Check sheet for the modelled part. Datum: model origin and axes. Units: mm. A direction names the side the tool comes from. Round coordinates to 2 decimals unless told otherwise and drop trailing zeros. Write each loop counter-clockwise with the first axis right and the second up, starting at its lowest first coordinate (ties: lowest second). Pieces come first, ordered by that corner, then holes. Notation, with made-up numbers: M -25.5,-40 L -11.5,-40 A8 cw -11.5,-29 Z; hole C 86.25,43 d8. An arc over 180 degrees is marked long. Put each result on its own line as item: value.
```python
from build123d import *

# Parameters (mm, degrees)
F1_R     = 1.5499996566
F1_R_2   = 4.15
F1_R_3   = 10.975
F2_DEPTH = 15
F3_R     = 1.5499996566
F3_R_2   = 10.975
F3_R_3   = 4.15
F3_R_4   = 5
F4_DEPTH = 8
F5_SIZE  = 0.5


# Not quite as in the source:
# - a feature names something its author has since deleted; it is built from what else it names


with BuildPart() as f2:
    # F1 (on offset) → F2 (new body)
    with BuildSketch(Plane.XZ.offset(7.5)):
        with BuildLine():
            ThreePointArc((-16.6892397333, 5.7083826769), (-18.3305665894, 4.8749174948), (-20.1713586703, 4.8647896648))
            ThreePointArc((-20.1713586703, 4.8647896648), (-26.2950827169, -0.0072979827), (-20.1713596113, -4.879386813))
            ThreePointArc((-20.1713596113, -4.879386813), (-18.3305675322, -4.8895149984), (-16.6892408371, -5.7229804975))
            ThreePointArc((-16.6892408371, -5.7229804975), (-14.008426037, -7.1768258733), (-10.9702112996, -7.4408061354))
            ThreePointArc((-10.9702112996, -7.4408061354), (-6.8485397196, -7.8126278343), (-3.2303605207, -9.8214103693))
            ThreePointArc((-3.2303605207, -9.8214103693), (7.2785660743, -12.855093715), (16.3833205976, -6.7933928076))
            ThreePointArc((16.3833205976, -6.7933928076), (18.1382514389, -5.2406931628), (20.4617514792, -4.9373682419))
            ThreePointArc((20.4617514792, -4.9373682419), (26.2950863861, -0.0073004118), (20.4617519197, 4.9227679396))
            ThreePointArc((20.4617519197, 4.9227679396), (18.1382519066, 5.2260930681), (16.383321204, 6.7787928697))
            ThreePointArc((16.383321204, 6.7787928697), (7.2785667206, 12.8404946682), (-3.2303604104, 9.8068115182))
            ThreePointArc((-3.2303604104, 9.8068115182), (-6.8485396319, 7.7980290238), (-10.970211216, 7.4262073712))
            ThreePointArc((-10.970211216, 7.4262073712), (-14.0084253044, 7.1622273392), (-16.6892397333, 5.7083826769))
        make_face()
        with Locations((21.2950848365, -0.0073001884)):
            Circle(F1_R, mode=Mode.SUBTRACT)
        with Locations((-21.2950828407, -0.0072984656)):
            Circle(F1_R, mode=Mode.SUBTRACT)
        with Locations((-11.8549144411, -0.0072993771)):
            Circle(F1_R_2, mode=Mode.SUBTRACT)
        with Locations((5.2950859535, -0.0072994735)):
            Circle(F1_R_3, mode=Mode.SUBTRACT)
    extrude(amount=-F2_DEPTH)

    # F3 (on face) → F4 (join)
    with BuildSketch(Plane(origin=(0, 7.5, 0), x_dir=(-1, 0, 0), z_dir=(0, 1, 0))):
        with BuildLine():
            ThreePointArc((10.970211216, 7.4262073712), (6.8485396319, 7.7980290238), (3.2303604104, 9.8068115182))
            ThreePointArc((3.2303604104, 9.8068115182), (-7.2785667206, 12.8404946682), (-16.383321204, 6.7787928697))
            ThreePointArc((-16.383321204, 6.7787928697), (-18.1382519066, 5.2260930681), (-20.4617519197, 4.9227679396))
            ThreePointArc((-20.4617519197, 4.9227679396), (-26.2950863861, -0.0073004118), (-20.4617514792, -4.9373682419))
            ThreePointArc((-20.4617514792, -4.9373682419), (-18.1382514389, -5.2406931628), (-16.3833205976, -6.7933928076))
            ThreePointArc((-16.3833205976, -6.7933928076), (-7.2785660743, -12.855093715), (3.2303605207, -9.8214103693))
            ThreePointArc((3.2303605207, -9.8214103693), (6.8485397196, -7.8126278343), (10.9702112996, -7.4408061354))
            ThreePointArc((10.9702112996, -7.4408061354), (14.008426037, -7.1768258733), (16.6892408371, -5.7229804975))
            ThreePointArc((16.6892408371, -5.7229804975), (18.3305675322, -4.8895149984), (20.1713596113, -4.879386813))
            ThreePointArc((20.1713596113, -4.879386813), (26.2950827169, -0.0072979827), (20.1713586703, 4.8647896648))
            ThreePointArc((20.1713586703, 4.8647896648), (18.3305665894, 4.8749174948), (16.6892397333, 5.7083826769))
            ThreePointArc((16.6892397333, 5.7083826769), (14.0084253044, 7.1622273392), (10.970211216, 7.4262073712))
        make_face()
        with Locations((-21.2950848365, -0.0073001884)):
            Circle(F3_R, mode=Mode.SUBTRACT)
        with Locations((-5.2950859535, -0.0072994735)):
            Circle(F3_R_2, mode=Mode.SUBTRACT)
        with Locations((11.8549144411, -0.0072993771)):
            Circle(F3_R_3, mode=Mode.SUBTRACT)
        with Locations((21.2950828407, -0.0072984656)):
            Circle(F3_R, mode=Mode.SUBTRACT)
        with Locations((-5.2950859535, -0.0072994735)):
            Circle(F3_R_2)
        with Locations((-5.2950859535, -0.0072994735)):
            Circle(F3_R_4, mode=Mode.SUBTRACT)
    extrude(amount=-F4_DEPTH)

    # F5
    f5_edges = [f2.edges().sort_by_distance(p)[0] for p in [
        (-6.84854, -7.5, 7.798029),
        (7.278567, -7.5, 12.840495),
        (18.138252, -7.5, 5.226093),
        (26.295086, -7.5, -0.0073),
        (18.138251, -7.5, -5.240693),
        (7.278566, -7.5, -12.855094),
        (-6.84854, -7.5, -7.812628),
        (-14.008426, -7.5, -7.176826),
        (-18.330568, -7.5, -4.889515),
        (-26.295083, -7.5, -0.007298),
        (-18.330567, -7.5, 4.874917),
        (-14.008425, -7.5, 7.162227),
        (-5.679914, -7.5, -0.007299),
        (-22.845082, -7.5, -0.007298),
        (19.745085, -7.5, -0.0073),
        (7.278567, 7.5, 12.840495),
        (-22.845082, 7.5, -0.007298),
        (10.295086, 7.5, -0.007299),
        (19.745085, 7.5, -0.0073),
        (-16.004914, -7.5, -0.007299),
        (-6.84854, 7.5, 7.798029),
        (-14.008425, 7.5, 7.162227),
        (-18.330567, 7.5, 4.874917),
        (-26.295083, 7.5, -0.007298),
        (-18.330568, 7.5, -4.889515),
        (-14.008426, 7.5, -7.176826),
        (-6.84854, 7.5, -7.812628),
        (7.278566, 7.5, -12.855094),
        (18.138251, 7.5, -5.240693),
        (26.295086, 7.5, -0.0073),
        (18.138252, 7.5, 5.226093),
    ]]
    chamfer(f5_edges, length=F5_SIZE)


solid = f2.part
```
1. Cross-section at C-C (y = 4.5). Enter the section's corners in (x, z).
Computed values:
outline: M -20.17,-4.88 A4 cw -16.69,-5.72 A7.49 ccw -10.97,-7.44 A10 cw -3.23,-9.82 A13 ccw 16.38,-6.79 A4 cw 20.46,-4.94 A5 ccw long 20.46,4.92 A4 cw 16.38,6.78 A13 ccw -3.23,9.81 A10 cw -10.97,7.43 A7.49 ccw -16.69,5.71 A4 cw -20.17,4.86 A5 ccw long Z; hole C -21.3,-0.01 d3.1; hole C -11.85,-0.01 d8.3; hole C 5.3,-0.01 d10; hole C 21.3,-0.01 d3.1
2. Scan lines: probe 1 along X at (y, z) = (1, -0.5); probe 2 along X at (y, z) = (-3.75, -2.5); probe 3 along Y at (x, z) = (-4.5, -2.25). Record each from-to range of solid material in increasing order.
Computed values:
probe 1: x = -26.27 to -22.76, -19.83 to -15.98, -7.73 to 0.32, 10.27 to 19.83, 22.76 to 26.27
probe 2: x = -25.63 to -15.17, -8.54 to -5.39, 15.98 to 25.63
probe 3: y = -0.5 to 7.5
3. Cross-section at A-A (y = -4). Enter the section's corners in (x, z) (3 decimals), then the cut area to 3 significant figures.
Computed values:
outline: M -20.171,-4.879 A4 cw -16.689,-5.723 A7.486 ccw -10.97,-7.441 A10 cw -3.23,-9.821 A13 ccw 16.383,-6.793 A4 cw 20.462,-4.937 A5 ccw long 20.462,4.923 A4 cw 16.383,6.779 A13 ccw -3.23,9.807 A10 cw -10.97,7.426 A7.486 ccw -16.689,5.708 A4 cw -20.171,4.865 A5 ccw long Z; hole C -21.295,-0.007 d3.1; hole C -11.855,-0.007 d8.3; hole C 5.295,-0.007 d21.95; hole C 21.295,-0.007 d3.1
area: 386 mm2
4. Cross-section at B-B (z = 2.75). Count the separate pieces of the cut face and the enclosed holes in it, then the cut area to 3 significant figures.
Computed values:
separate pieces: 3
enclosed holes: 0
area: 454 mm2
5. Access from +Z, -Z, +X, -X, +Y, -Y to the whole of each face (thin tool, end or side, straight path). Record for faces 1 (the cylindrical face through (-26.293, -0.098, 0.119)), 2 (the flat face through (0.6, -0.5, -2.3)).
Computed values:
face 1: +Y, -Y
face 2: -Y
6. Depth check by flat-ended pin: pin 1 Ø11 at (x, z) = (-11.85, -0.01) entering from -Y; pin 2 Ø1.5 at (y, z) = (-4.5, 10) entering from -X; pin 3 Ø6 at (y, z) = (-5.5, -5) entering from +X; pin 4 Ø4 at (x, y) = (18.5, 0.5) entering from +Z. Enter the tip coordinate at first touch or a pass-through.
Computed values:
pin 1: stops at y = -7.5
pin 2: stops at x = -3.93
pin 3: stops at x = 25.88
pin 4: stops at z = 6.6
